```python
from build123d import *

# Parameters (mm, degrees)
SKETCH1_R           = 16.51
SKETCH1_R_2         = 6.35
BOSS_EXTRUDE1_DEPTH = 3.175
CIRPATTERN1_COUNT   = 4
SKETCH4_R           = 0.635
CUT_EXTRUDE1_DEPTH  = 3.175
CIRPATTERN2_COUNT   = 15


with BuildPart() as part:
    # Sketch1 → Boss-Extrude1 (new body)
    with BuildSketch(Plane(origin=(0, 0, 0), x_dir=(1, 0, 0), z_dir=(0, 1, 0))):
        Circle(SKETCH1_R)
        Circle(SKETCH1_R_2, mode=Mode.SUBTRACT)
    extrude(amount=BOSS_EXTRUDE1_DEPTH)

    # Sketch2 → #4 Clearance Hole1 (revolve, cut)
    with BuildSketch(Plane(origin=(0, 3.175, -10.16), x_dir=(0, 0, 1), z_dir=(1, 0, 0))):
        Polygon((0, 0), (0, 11.140574487), (1.63195, 10.16), (1.63195, 0), align=None)
    f_4_clearance_hole1 = revolve(axis=Axis((0, 9.525, -10.16), (0, -1, 0)), mode=Mode.SUBTRACT)

    # CirPattern1: #4 Clearance Hole1 ×4 about axis
    cirpattern1_axis = Axis((0, 0, 0), (0, 1, 0))
    for i in range(1, CIRPATTERN1_COUNT):
        add(f_4_clearance_hole1.rotate(cirpattern1_axis, i * 360 / CIRPATTERN1_COUNT), mode=Mode.SUBTRACT)

    # Sketch4 → Cut-Extrude1 (cut)
    with BuildSketch(Plane(origin=(0, 3.175, 0), x_dir=(1, 0, 0), z_dir=(0, 1, 0))):
        with Locations((0, 15.24)):
            Circle(SKETCH4_R)
    cut_extrude1 = extrude(amount=-CUT_EXTRUDE1_DEPTH, mode=Mode.SUBTRACT)

    # CirPattern2: Cut-Extrude1 ×15 about axis
    cirpattern2_axis = Axis((0, 0, 0), (0, 1, 0))
    for i in range(1, CIRPATTERN2_COUNT):
        add(cut_extrude1.rotate(cirpattern2_axis, i * 360 / CIRPATTERN2_COUNT), mode=Mode.SUBTRACT)


solid = part.part
```
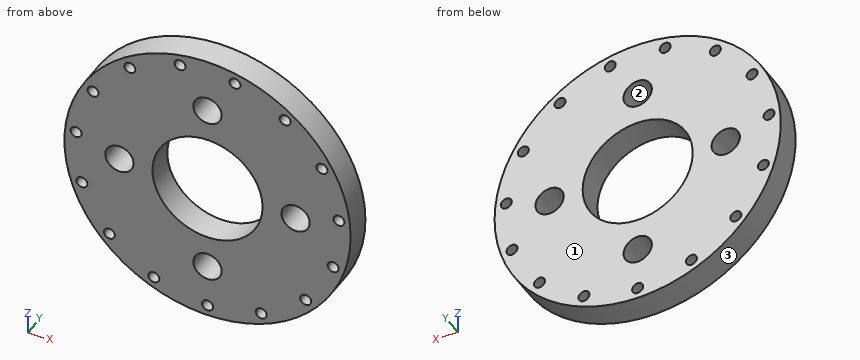
Here's how the part is built. I have some questions about the finished solid (model axes, mm). Face numbers are marked on the shaded views. Coordinates: 2 decimals unless noted, no trailing zeros. Order: outer loops, then holes, each group sorted by start corner. A loop starts at its lowest first (then second) coordinate and runs counter-clockwise, first axis right, second up.
Item 1: If we section it at A-A, the plane z = 10.16: List the corners of the cut face in (x, y) for me (3 decimals), then the cut area to 3 significant figures.
Response values:
outline: (-13.014, 0) - (-1.632, 0) - (-1.632, 3.175) - (-13.014, 3.175) - close; (1.632, 0) - (13.014, 0) - (13.014, 3.175) - (1.632, 3.175) - close
area: 72.3 mm2
Item 2: If we section it at C-C, the plane z = 0.5: List the corners of the cut face in (x, y) for me (3 decimals).
Response values:
outline: (-16.502, 0) - (-11.713, 0) - (-11.713, 3.175) - (-16.502, 3.175) - close; (-8.607, 0) - (-6.33, 0) - (-6.33, 3.175) - (-8.607, 3.175) - close; (6.33, 0) - (8.607, 0) - (8.607, 3.175) - (6.33, 3.175) - close; (11.713, 0) - (16.502, 0) - (16.502, 3.175) - (11.713, 3.175) - close
Item 3: I'm going to push flat-ended pins straight in: pin 1 Ø3 at (x, z) = (-10.16, 0) entering from -Y; pin 2 Ø1.5 at (x, z) = (6.2, -13.92) entering from +Y (3 decimals); pin 3 Ø1 at (y, z) = (2.5, 5) entering from -X. Where does each tip first touch, or does it pass through?
Response values:
pin 1: passes through
pin 2: stops at y = 3.175
pin 3: stops at x = -15.88
Item 4: Thinking about a two-plate mould opening in X: for the marked faces 1, 2 and 3, which applies, pulls with the +X half, pulls with the -X half, needs draft (parallel to the pull), parting line crosses it, or undercut?
Response values:
face 1: needs draft
face 2: undercut
face 3: parting line crosses it
Item 5: If we section it at B-B, the plane x = -10.16: List the corners of the cut face in (y, z) for me (3 decimals), then the cut area to 3 significant figures.
Response values:
outline: (0, -13.014) - (3.175, -13.014) - (3.175, -1.632) - (0, -1.632) - close; (0, 1.632) - (3.175, 1.632) - (3.175, 13.014) - (0, 13.014) - close
area: 72.3 mm2
Item 6: If we section it at D-D, the plane y = 2.7: Give the number of separate pieces and of enclosed holes in the cut face, then the cut area to 3 significant figures.
Response values:
separate pieces: 1
enclosed holes: 20
area: 677 mm2
Item 7: I need wall thicknesses on probe 1 along Z at (x, y) = (0, 2) (3 decimals); probe 2 along Z at (x, y) = (3, 0.8); probe 3 along X at (y, z) = (1.15, -1). Which ranges of each line are inside material? Lowest first, please.
Response values:
probe 1: z = -16.51 to -15.875, -14.605 to -11.792, -8.528 to -6.35, 6.35 to 8.528, 11.792 to 16.51
probe 2: z = -16.24 to -5.6, 5.6 to 14.29, 15.52 to 16.24
probe 3: x = -16.48 to -11.45, -8.87 to -6.27, 6.27 to 8.87, 11.45 to 16.48
